For this review, take the finished solid that the model builds, in its own axes (mm). Face numbers are marked on the shaded views. A direction names the side the tool comes from. Give positions to 0.01 mm unless a question says otherwise; leave off trailing zeros. Write each loop counter-clockwise with the first axis right and the second up, starting at its lowest first coordinate (ties: lowest second). Pieces come first, ordered by that corner, then holes.
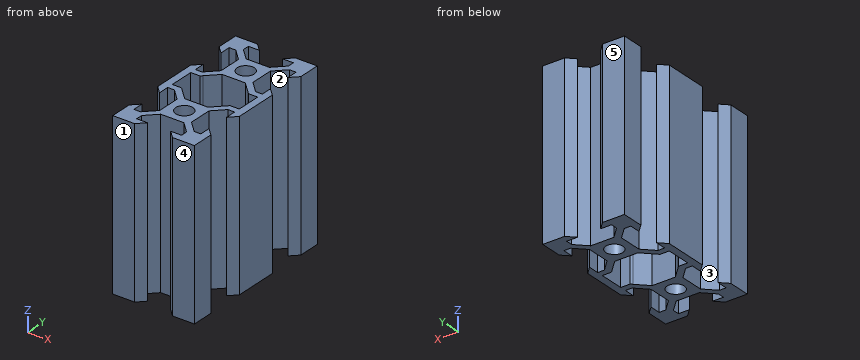
Autodesk Inventor part; units mm, degrees
ref_plane "Work Plane3" through (0, -20, 0) normal (0, 1, 0) x (-1, 0, 0)
ref_plane "YZ Plane" through (0, 0, 0) normal (1, 0, 0) x (0, 1, 0)
ref_plane "XY Plane" through (0, 0, 0) normal (0, 0, 1) x (1, 0, 0)
sketch "Sketch1" plane through (0, 0, 0) normal (0, 0, 1) x (1, 0, 0)
  line L0 (-3.9007, 3.9007) -> (3.9007, 3.9007)
  line L1 (3.9007, 3.9007) -> (3.9007, -3.9007)
  line L2 (3.9007, -3.9007) -> (-3.9007, -3.9007)
  line L3 (-3.9007, -3.9007) -> (-3.9007, 3.9007)
  line L4 (0, 3.9007) -> (0, -3.9007) construction
  line L5 (-3.9007, 0) -> (3.9007, 0) construction
  circle A0 centre (0, 0) radius 2.1
  line L6 (0, 0) -> (-16.1173, 16.1173) construction
  line L7 (0, 0) -> (22.7933, 0) construction
  line L8 (-2.84, 3.9007) -> (-5.4993, 6.56)
  line L9 (-5.4993, 6.56) -> (-5.4993, 8.2)
  line L10 (-5.4993, 8.2) -> (-2.84, 8.2)
  line L11 (-2.84, 8.2) -> (-4.64, 10)
  line L12 (-4.64, 10) -> (-10, 10)
  line L13 (-10, 10) -> (-10, 4.64)
  line L14 (-10, 4.64) -> (-8.2, 2.84)
  line L15 (-8.2, 2.84) -> (-8.2, 5.4993)
  line L16 (-8.2, 5.4993) -> (-6.56, 5.4993)
  line L17 (-6.56, 5.4993) -> (-3.9007, 2.84)
  line L18 (-3.9007, 2.84) -> (-11.3102, 2.84) construction
  line L19 (-2.84, 3.9007) -> (-3.9007, 3.9007)
  line L20 (-3.9007, 2.84) -> (-3.9007, 3.9007)
  line L21 (-3.9007, -2.84) -> (-6.56, -5.4993)
  line L22 (-6.56, -5.4993) -> (-8.2, -5.4993)
  line L23 (-8.2, -5.4993) -> (-8.2, -2.84)
  line L24 (-8.2, -2.84) -> (-10, -4.64)
  line L25 (-10, -4.64) -> (-10, -10)
  line L26 (-10, -10) -> (-4.64, -10)
  line L27 (-4.64, -10) -> (-2.84, -8.2)
  line L28 (-2.84, -8.2) -> (-5.4993, -8.2)
  line L29 (-5.4993, -8.2) -> (-5.4993, -6.56)
  line L30 (-5.4993, -6.56) -> (-2.84, -3.9007)
  line L31 (-3.9007, -2.84) -> (-3.9007, -3.9007)
  line L32 (-2.84, -3.9007) -> (-3.9007, -3.9007)
  line L33 (2.84, -3.9007) -> (5.4993, -6.56)
  line L34 (5.4993, -6.56) -> (5.4993, -8.2)
  line L35 (5.4993, -8.2) -> (2.84, -8.2)
  line L36 (2.84, -8.2) -> (4.64, -10)
  line L37 (4.64, -10) -> (10, -10)
  line L38 (10, -10) -> (10, -4.64)
  line L39 (10, -4.64) -> (8.2, -2.84)
  line L40 (8.2, -2.84) -> (8.2, -5.4993)
  line L41 (8.2, -5.4993) -> (6.56, -5.4993)
  line L42 (6.56, -5.4993) -> (3.9007, -2.84)
  line L43 (2.84, -3.9007) -> (3.9007, -3.9007)
  line L44 (3.9007, -2.84) -> (3.9007, -3.9007)
  line L45 (3.9007, 2.84) -> (6.56, 5.4993)
  line L46 (6.56, 5.4993) -> (8.2, 5.4993)
  line L47 (8.2, 5.4993) -> (8.2, 2.84)
  line L48 (8.2, 2.84) -> (10, 4.64)
  line L49 (10, 4.64) -> (10, 10)
  line L50 (10, 10) -> (4.64, 10)
  line L51 (4.64, 10) -> (2.84, 8.2)
  line L52 (2.84, 8.2) -> (5.4993, 8.2)
  line L53 (5.4993, 8.2) -> (5.4993, 6.56)
  line L54 (5.4993, 6.56) -> (2.84, 3.9007)
  line L55 (3.9007, 2.84) -> (3.9007, 3.9007)
  line L56 (2.84, 3.9007) -> (3.9007, 3.9007)
  dimension "d7" = 4.2
  dimension "d8" = 135
  dimension "d9" = 1.5
  dimension "d10" = 1.64
  dimension "d11" = 1.8
  dimension "d12" = 2.84
  dimension "d13" = 10
  dimension "d16" = 360
extrude "Extrusion1" add sketch "Sketch1" along normal blind 40
pattern_linear "Rectangular Pattern1" count 2 spacing 20 along (0, -1, 0) of "Extrusion1"
sketch "Sketch2" plane through (0, 0, 40) normal (0, 0, 1) x (1, 0, 0)
  line L0 (8.2, -2.84) -> (8.2, -5.4993)
  line L1 (8.2, -5.4993) -> (6.56, -5.4993)
  line L2 (-6.56, -5.4993) -> (-8.2, -5.4993)
  line L3 (-8.2, -5.4993) -> (-8.2, -2.84)
  line L4 (-8.2, -14.5007) -> (-6.56, -14.5007)
  line L5 (6.56, -14.5007) -> (8.2, -14.5007)
  line L6 (5.4993, -11.8) -> (5.4993, -13.44)
  line L7 (5.4993, -13.44) -> (2.84, -16.0993)
  line L8 (-2.84, -16.0993) -> (-5.4993, -13.44)
  line L9 (-5.4993, -8.2) -> (-5.4993, -6.56)
  line L10 (-5.4993, -6.56) -> (-2.84, -3.9007)
  line L11 (2.84, -3.9007) -> (5.4993, -6.56)
  line L12 (2.84, -8.2) -> (4.64, -10)
  line L13 (-8.2, -6.9993) -> (-5.9387, -6.9993)
  line L14 (-5.9387, -6.9993) -> (-4.1231, -5.1837)
  line L15 (-4.1231, -5.1837) -> (4.1231, -5.1837)
  line L16 (4.1231, -5.1837) -> (5.9387, -6.9993)
  line L17 (5.9387, -6.9993) -> (8.2, -6.9993)
  line L18 (8.2, -6.9993) -> (8.2, -13.0007)
  line L19 (8.2, -13.0007) -> (5.9387, -13.0007)
  line L20 (5.9387, -13.0007) -> (4.2461, -14.6932)
  line L21 (4.2461, -14.6932) -> (-4.2461, -14.6932)
  line L22 (-4.2461, -14.6932) -> (-5.9387, -13.0007)
  line L23 (-5.9387, -13.0007) -> (-8.2, -13.0007)
  line L24 (-8.2, -13.0007) -> (-8.2, -6.9993)
  dimension "d23" = 1.5
  dimension "d24" = 1.5
  dimension "d25" = 1.5
  dimension "d26" = 1.5
extrude "Extrusion2" cut sketch "Sketch2" against normal up to next
ref_plane "Work Plane3" through (0, -20, 0) normal (0, 1, 0) x (-1, 0, 0)
ref_plane "Work Plane2" through (0, 0, 0) normal (0, 1, 0) x (-1, 0, 0)
ref_plane "Work Plane1" through (0, -10, 0) normal (0, 1, 0) x (-1, 0, 0)
equation "\"d24\" = d23"
equation "\"d25\" = d23"
equation "\"d26\" = d23"
properties part number "20x40x597mm" material "Aluminum 6061"
(1) The part is to be moulded in two halves that separate along Y. For the marked faces 3, 4 and 5, say which applies: +Y half, -Y half, draft (parallel to the pull), parting line (faces both ways), or undercut.
(2) We need section A-A (y = 0). Write out the cut boundary in (x, z), and give its area (3 significant figures).
(3) Tool access review of the marked faces 1 and 2: name each direction out of +Z, -Z, +X, -X, +Y, -Y from which nothing blocks a thin tool from reaching the whole face with its end or side.
(4) We need section C-C (y = -19). Write out the cut boundary in (x, z), and give its area (3 significant figures).
(5) For L1, parallel to Y at x = 7.5, z = 27.5; L2, parallel to Y at x = 0, z = 30; L3, parallel to Y at x = -4, z = 37.5, list the stretches that pass through material, from the lowest coordinate up.
(6) We need section D-D (z = 23). Count the separate pieces of the cut face and the enclosed holes in it, and give its area (3 significant figures).
(7) We need section B-B (x = 0). Write out the cut boundary in (y, z), and give its area (3 significant figures).
(8) Clearance check with flat-ended pins moving along their axes: pin 1 Ø4.5 at (y, z) = (0, 25.5) entering from +X; pin 2 Ø1.7 at (y, z) = (0, 29) entering from -X; pin 3 Ø4.5 at (x, z) = (-0.5, 17.5) entering from -Y. State where each tip first meets the part, or that it passes through.
The answers:
1. face 3: undercut
1. face 4: -Y half
1. face 5: +Y half
2. outline: (-3.9, 0) - (-2.1, 0) - (-2.1, 40) - (-3.9, 40) - close; (2.1, 0) - (3.9, 0) - (3.9, 40) - (2.1, 40) - close
2. area: 144 mm2
3. face 1: +Z, -Z, +X, -X, -Y
3. face 2: +Z, -Z
4. outline: (-3.9, 0) - (-1.85, 0) - (-1.85, 40) - (-3.9, 40) - close; (1.85, 0) - (3.9, 0) - (3.9, 40) - (1.85, 40) - close
4. area: 164 mm2
5. L1: y = -30 to -25.5, -14.5 to -13, -7 to -5.5, 5.5 to 10
5. L2: y = -23.9 to -22.1, -17.9 to -16.1, -3.9 to -2.1, 2.1 to 3.9
5. L3: y = -29.36 to -28.2, -25.06 to -22.94, -17.06 to -14.94, -5.06 to -2.94, 2.94 to 5.06, 8.2 to 9.36
6. separate pieces: 1
6. enclosed holes: 3
6. area: 297 mm2
7. outline: (-23.9, 0) - (-22.1, 0) - (-22.1, 40) - (-23.9, 40) - close; (-17.9, 0) - (-16.1, 0) - (-16.1, 40) - (-17.9, 40) - close; (-3.9, 0) - (-2.1, 0) - (-2.1, 40) - (-3.9, 40) - close; (2.1, 0) - (3.9, 0) - (3.9, 40) - (2.1, 40) - close
7. area: 288 mm2
8. pin 1: stops at x = 3.9
8. pin 2: stops at x = -3.9
8. pin 3: stops at y = -23.9
